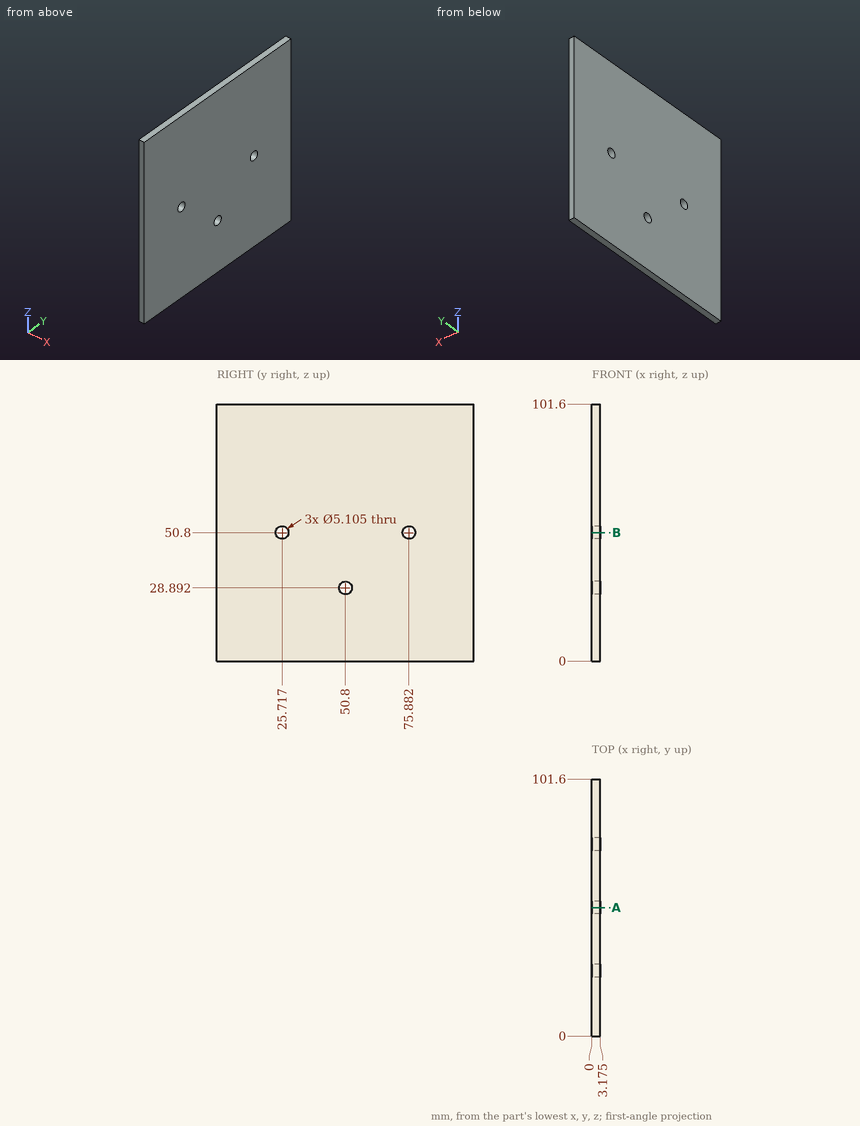
Check sheet for the drawn part. Datum: minimum x, y, z corner. Units: mm. Give positions to 0.01 mm unless a question says otherwise; leave off trailing zeros. Write each loop counter-clockwise with the first axis right and the second up, starting at its lowest first coordinate (ties: lowest second). Pieces come first, ordered by that corner, then holes. Notation, with made-up numbers: (16.5, 8) - (31.5, 8) arc R12 cw to (31.5, 12) - close; hole circle Ø10 at (-37, 67). An arc over 180 degrees is marked (long way). Put each result on its own line as item: value.
1. Go/stop test with a flat-tipped pin: pin 1 (4.5 mm diameter, centred on y = 50.8, z = 28.89, fed in from +X). Record where the tip stops, or that it passes through.
Ans:
pin 1: passes through
2. Thickness scan on line 1 (Y direction, x = 0.6, z = 49.5) (1 decimal); line 2 (Z direction, x = 1.75, y = 50.5); line 3 (Z direction, x = 2.75, y = 24). Record the ranges inside material, lowest first.
Ans:
line 1: y = 0 to 23.5, 27.9 to 73.7, 78.1 to 101.6
line 2: z = 0 to 26.36, 31.43 to 101.6
line 3: z = 0 to 48.91, 52.69 to 101.6
3. Sectioned sample at B-B, the plane z = 50.8. Enter the section's corners in (x, y) (1 decimal).
Ans:
outline: (0, 0) - (3.2, 0) - (3.2, 23.2) - (0, 23.2) - close; (0, 28.3) - (3.2, 28.3) - (3.2, 73.3) - (0, 73.3) - close; (0, 78.4) - (3.2, 78.4) - (3.2, 101.6) - (0, 101.6) - close
4. Sectioned sample at A-A, the plane y = 50.8. Enter the section's corners in (x, z) (1 decimal).
Ans:
outline: (0, 0) - (3.2, 0) - (3.2, 26.3) - (0, 26.3) - close; (0, 31.4) - (3.2, 31.4) - (3.2, 101.6) - (0, 101.6) - close
